CAD build for the part. Positions are in the model's coordinates, mm. Round coordinates to 2 decimals unless told otherwise and drop trailing zeros. Write each loop counter-clockwise with the first axis right and the second up, starting at its lowest first coordinate (ties: lowest second). Pieces come first, ordered by that corner, then holes. Notation, with made-up numbers: M 55,46.25 L 109,46.25 A19 ccw 109,83.25 Z; hole C -20,-26.75 d2. An arc over 180 degrees is marked long. Write each question's results on one line, items separated by ' | '. Start each with the question number.
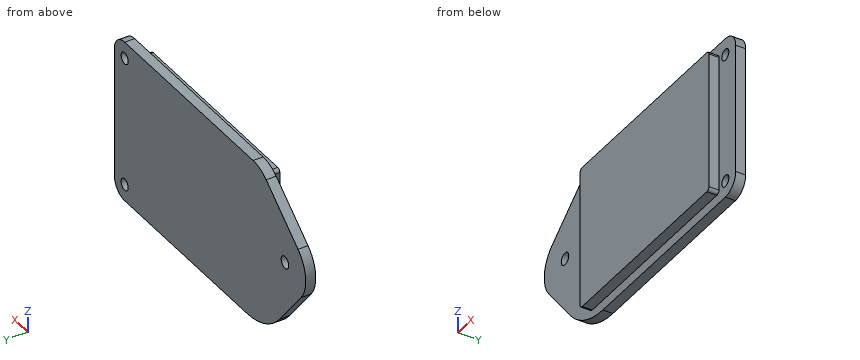
```python
from build123d import *

# Parameters (mm, degrees)
SKETCH1_R           = 1.7
BOSS_EXTRUDE2_DEPTH = 3
BOSS_EXTRUDE3_DEPTH = 3
SKETCH4_R           = 1.8
CUT_EXTRUDE1_DEPTH  = 5


with BuildPart() as part:
    # Sketch1 → Boss-Extrude2 (new body)
    with BuildSketch(Plane(origin=(0, 0, 0), x_dir=(1, 0, 0), z_dir=(0, 1, 0))):
        with BuildLine():
            Line((-39.007261737, -39.092855818), (22.832898339, -39.092855818))
            ThreePointArc((22.832898339, -39.092855818), (26.368432245, -37.628389724), (27.832898339, -34.092855818))
            Line((27.832898339, -34.092855818), (27.832898339, 4.907144182))
            ThreePointArc((27.832898339, 4.907144182), (26.368432245, 8.442678088), (22.832898339, 9.907144182))
            Line((22.832898339, 9.907144182), (-36.143461968, 9.907144182))
            ThreePointArc((-36.143461968, 9.907144182), (-44.75263802, 7.959348694), (-51.684922644, 2.495352954))
            Line((-51.684922644, 2.495352954), (-62.112298102, -10.378332935))
            ThreePointArc((-62.112298102, -10.378332935), (-64.286907773, -17.716569545), (-60.63567215, -24.443167658))
            Line((-60.63567215, -24.443167658), (-45.301366123, -36.863586155))
            ThreePointArc((-45.301366123, -36.863586155), (-42.345876466, -38.519077314), (-39.007261737, -39.092855818))
        make_face()
        with Locations(Location((22.832898339, 4.907144182, 0), (0, 0, 270))):
            Circle(SKETCH1_R, mode=Mode.SUBTRACT)
        with Locations(Location((22.832898339, -34.092855818, 0), (0, 0, 270))):
            Circle(SKETCH1_R, mode=Mode.SUBTRACT)
    extrude(amount=BOSS_EXTRUDE2_DEPTH)

    # Sketch3 → Boss-Extrude3 (add)
    with BuildSketch(Plane.XZ):
        with BuildLine():
            ThreePointArc((-41.216654954, -6.9270495), (-41.923761735, -6.634156281), (-42.216654954, -5.9270495))
            Line((-42.216654954, -5.9270495), (-42.216654954, 35.0729505))
            ThreePointArc((-42.216654954, 35.0729505), (-41.923761735, 35.780057281), (-41.216654954, 36.0729505))
            Line((-41.216654954, 36.0729505), (18.783345046, 36.0729505))
            ThreePointArc((18.783345046, 36.0729505), (19.490451827, 35.780057281), (19.783345046, 35.0729505))
            Line((19.783345046, 35.0729505), (19.783345046, -5.9270495))
            ThreePointArc((19.783345046, -5.9270495), (19.490451827, -6.634156281), (18.783345046, -6.9270495))
            Line((18.783345046, -6.9270495), (-41.216654954, -6.9270495))
        make_face()
    extrude(amount=BOSS_EXTRUDE3_DEPTH)

    # Sketch4 → Cut-Extrude1 (cut)
    with BuildSketch(Plane(origin=(0, 3, 0), x_dir=(1, 0, 0), z_dir=(0, 1, 0))):
        with Locations(Location((-54.341567764, -16.672437321, 0), (0, 0, 270))):
            Circle(SKETCH4_R)
    extrude(amount=-CUT_EXTRUDE1_DEPTH, mode=Mode.SUBTRACT)


solid = part.part
```
1) Wall check: line 1 along Y through (x, z) = (-42.5, 0); line 2 along X through (y, z) = (0.05, 31); line 3 along Z through (x, y) = (-1, -0.55). Give the ranges that are in metal, low to high. Write a range as from..to.
2) Saw through at C-C, the plane z = 13. Write the cut outline in (x, y), plus the area to 3 significant figures.
3) Saw through at B-B, the plane y = 1.65. Write the cut outline in (x, z), plus the area to 3 significant figures.
4) Drop flat-ended pins along their axis: pin 1 Ø1.5 at (y, z) = (-1, 19) entering from +X; pin 2 Ø1 at (y, z) = (2, 5) entering from -X; pin 3 Ø3.5 at (x, y) = (-5.5, -2) entering from -Z. Give the stop position or say it passes through.
5) Saw through at A-A, the plane x = -7.5. Write the cut outline in (y, z), plus the area to 3 significant figures.
Filled sheet:
1) line 1: y = 0..3 | line 2: x = -52.54..27.83 | line 3: z = -6.93..36.07
2) outline: M -63.64,0 L -42.22,0 L -42.22,-3 L 19.78,-3 L 19.78,0 L 27.83,0 L 27.83,3 L -63.64,3 Z | area: 460 mm^2
3) outline: M -62.11,10.38 L -51.68,-2.5 A20 ccw -36.14,-9.91 L 22.83,-9.91 A5 ccw 27.83,-4.91 L 27.83,34.09 A5 ccw 22.83,39.09 L -39.01,39.09 A10 ccw -45.3,36.86 L -60.64,24.44 A10 ccw Z; hole C -54.34,16.67 d3.6; hole C 22.83,-4.91 d3.4; hole C 22.83,34.09 d3.4 | area: 4,050 mm^2
4) pin 1: stops at x = 19.78 | pin 2: stops at x = -58.16 | pin 3: stops at z = -6.93
5) outline: M -3,-6.93 L 0,-6.93 L 0,-9.91 L 3,-9.91 L 3,39.09 L 0,39.09 L 0,36.07 L -3,36.07 Z | area: 276 mm^2
